Check sheet for the modelled part. Datum: model origin and axes. Units: mm. A direction names the side the tool comes from. Round coordinates to 2 decimals unless told otherwise and drop trailing zeros. Loops run counter-clockwise (first coordinate to the right, second up) from the corner with the lowest first, then second, coordinate; pieces in that order, holes last. Notation, with made-up numbers: (84.25, 42) -> (120.25, 42) arc R17 ccw to (120.25, 72) -> close; hole circle Ø10 at (34.25, 55). An arc over 180 degrees is marked (long way). Return JSON: item names as keys, results as strings.
from build123d import *

# Parameters (mm, degrees)
F0_W     = 45
F0_H     = 55
F1_DEPTH = 10
F2_W     = 45
F2_H     = 10
F3_DEPTH = 30
F4_W     = 12
F4_H     = 10
F5_DEPTH = 10
F7_D     = 12
F7_DEPTH = 16
F9_D     = 6.5
F9_DEPTH = 10


with BuildPart() as f1:
    # F0 (on Front) → F1 (new body)
    with BuildSketch(Plane.XZ):
        Rectangle(F0_W, F0_H)
    extrude(amount=F1_DEPTH)

    # F2 (on face) → F3 (join)
    with BuildSketch(Plane.XZ.offset(10)):
        with Locations((0, -22.5)):
            Rectangle(F2_W, F2_H)
    extrude(amount=F3_DEPTH)

    # F4 (on face) → F5 (cut)
    with BuildSketch(Plane.XZ.offset(10)):
        with Locations((0, 12.5)):
            Rectangle(F4_W, F4_H)
    extrude(amount=-F5_DEPTH, mode=Mode.SUBTRACT)

    # F7
    with Locations(Plane.XZ.offset(10)):
        with Locations((0, 17.5), (0, 7.5)):
            Hole(F7_D / 2, depth=F7_DEPTH)

    # F9
    with Locations(Plane(origin=(0, 0, -27.5), x_dir=(1, 0, 0), z_dir=(0, 0, -1))):
        with Locations((-12.5, 20), (12.5, 20)):
            Hole(F9_D / 2, depth=F9_DEPTH)


solid = f1.part
Q1. Section check D-D (z = -19.5). Record the boundary of the cut face in (x, y).
Results list:
{"outline": "(-22.5, -40) -> (22.5, -40) -> (22.5, 0) -> (-22.5, 0) -> close; hole circle Ø6.5 at (-12.5, -20); hole circle Ø6.5 at (12.5, -20)"}
Q2. Go/stop test with flat-tipped pins: pin 1 (7.5 mm diameter, centred on x = 12.5, y = -20, fed in from -Z); pin 2 (10 mm diameter, centred on x = 9, z = 17, fed in from -Y); pin 3 (6 mm diameter, centred on x = -12.5, y = -20, fed in from -Z). Record where each tip stops, or that it passes through.
Results list:
{"pin 1": "z = -27.5", "pin 2": "y = -10", "pin 3": "through"}
Q3. Section check B-B (z = 10.5). Record the boundary of the cut face in (x, y), then the cut area to 3 significant figures.
Results list:
{"outline": "(-22.5, -10) -> (-6, -10) -> (-6, 0) -> (-22.5, 0) -> close; (6, -10) -> (22.5, -10) -> (22.5, 0) -> (6, 0) -> close", "area": "330 mm^2"}
Q4. Section check C-C (y = -20). Record the boundary of the cut face in (x, z).
Results list:
{"outline": "(-22.5, -27.5) -> (-15.75, -27.5) -> (-15.75, -17.5) -> (-22.5, -17.5) -> close; (-9.25, -27.5) -> (9.25, -27.5) -> (9.25, -17.5) -> (-9.25, -17.5) -> close; (15.75, -27.5) -> (22.5, -27.5) -> (22.5, -17.5) -> (15.75, -17.5) -> close"}
Q5. Section check A-A (x = 0). Record the boundary of the cut face in (y, z), then the cut area to 3 significant figures.
Results list:
{"outline": "(-40, -27.5) -> (0, -27.5) -> (0, 1.5) -> (-10, 1.5) -> (-10, -17.5) -> (-40, -17.5) -> close; (-10, 23.5) -> (0, 23.5) -> (0, 27.5) -> (-10, 27.5) -> close", "area": "630 mm^2"}
Q6. Material ranges on line 1 (X direction, y = -20, z = -21.25); line 2 (Y direction, x = -12.5, z = -23.75); line 3 (X direction, y = -7, z = 8.5), recorded low to high.
Results list:
{"line 1": "-22.5 to -15.75, -9.25 to 9.25, 15.75 to 22.5", "line 2": "-40 to -23.25, -16.75 to 0", "line 3": "-22.5 to -6, 6 to 22.5"}
Q7. Tool access check on faces 1 (the flat face through (0, -25, -17.5)), 2 (the flat face through (0, -5, 27.5)), 3 (the cylindrical face through (0.1, -4.9, 1.5)). Record the directions out of +Z, -Z, +X, -X, +Y, -Y that give a thin tool (end or side, any length) a straight path to the whole face; none if there is none.
Results list:
{"face 1": "+Z, +X, -X, -Y", "face 2": "+Z, +X, -X, +Y, -Y", "face 3": "+Y, -Y"}
Q8. Draft check along Y on faces 4 (the flat face through (0, -20, -27.5)), 5 (the cylindrical face through (15.079, -18.022, -22.43)), 6 (the flat face through (0, 0, 0)), 7 (the flat face through (0, -10, 0)). Enter one of: released by +Y, released by -Y, zero draft, split by the parting line, or undercut.
Results list:
{"face 4": "zero draft", "face 5": "undercut", "face 6": "released by +Y", "face 7": "released by -Y"}
